For this review, take the finished solid that the model builds, in its own axes (mm). A direction names the side the tool comes from. Give positions to 0.01 mm unless a question says otherwise; leave off trailing zeros. Loops run counter-clockwise (first coordinate to the right, second up) from the corner with the lowest first, then second, coordinate; pieces in that order, holes last. Notation, with made-up numbers: (49.5, 68.25) -> (71.5, 68.25) arc R29 ccw to (71.5, 100.25) -> close; hole circle Ø9 at (-2.75, 47). An arc over 180 degrees is marked (long way). One line per question, with ' | ' between items. Start each with the question number.
(1) Consider section A-A (y = -4). Write out the cut boundary in (x, z), and give its area (3 significant figures).
(2) Wall thickness on probe 1 along Z at (x, y) = (3.5, 1.5); probe 2 along Y at (x, z) = (-4, 4.5); probe 3 along X at (y, z) = (0.75, 12.25): over which ranges is each line inside the solid? List them lowest first.
(3) Consider section C-C (z = 14.5). Write out the cut boundary in (x, y), and give its area (3 significant figures).
(4) Insertion check: P1, Ø5, axis at x = -4, z = 4.5, coming from the -Y side; P2, Ø1, axis at x = 2, z = 2, coming from the +Y side; P3, Ø5, axis at y = -3, z = 7, coming from the -X side. Each pin has a flat end and moves straight along its axis. Give the tip position at first contact, or say it passes through.
(5) Consider section B-B (x = -4.5). Write out the cut boundary in (y, z), and give its area (3 significant figures).
(6) Consider section D-D (x = 0). Write out the cut boundary in (y, z), and give its area (3 significant figures).
(7) Draft analysis for pull direction Z (two halves, no side actions). For faces 1 (the flat face through (-0.1, -3.3, 5)), 2 (the flat face through (0, 0, 0)), 3 (the cylindrical face through (-7.4, 0, 1.5)), state which applies: +Z half, -Z half, draft (parallel to the pull), parting line (faces both ways), or undercut.
(8) Tool access review of faces 4 (the cylindrical face through (-3, 0, 7)), 5 (the flat face through (0, 0, 18)): name each direction out of +Z, -Z, +X, -X, +Y, -Y from which nothing blocks a thin tool from reaching the whole face with its end or side.
from build123d import *

# Parameters (mm, degrees)
SKETCH2_R           = 5
BOSS_EXTRUDE1_DEPTH = 5
SKETCH3_R           = 3
BOSS_EXTRUDE2_DEPTH = 5
SKETCH4_R           = 5
BOSS_EXTRUDE3_DEPTH = 8
SKETCH5_R           = 1
BOSS_EXTRUDE4_DEPTH = 10


with BuildPart() as part:
    # Sketch2 → Boss-Extrude1 (new body)
    with BuildSketch(Plane.XY):
        Circle(SKETCH2_R)
    extrude(amount=BOSS_EXTRUDE1_DEPTH)

    # Sketch3 → Boss-Extrude2 (add)
    with BuildSketch(Plane.XY.offset(5)):
        Circle(SKETCH3_R)
    extrude(amount=BOSS_EXTRUDE2_DEPTH)

    # Sketch4 → Boss-Extrude3 (add)
    with BuildSketch(Plane.XY.offset(10)):
        Circle(SKETCH4_R)
    extrude(amount=BOSS_EXTRUDE3_DEPTH)

    # Sketch5 → Boss-Extrude4 (add)
    with BuildSketch(Plane.ZY):
        with Locations((2.5, 0)):
            Circle(SKETCH5_R)
    extrude(amount=BOSS_EXTRUDE4_DEPTH)


solid = part.part
A:
1) outline: (-3, 0) -> (3, 0) -> (3, 5) -> (-3, 5) -> close; (-3, 10) -> (3, 10) -> (3, 18) -> (-3, 18) -> close | area: 78.0 mm^2
2) probe 1: z = 0 to 5, 10 to 18 | probe 2: y = -3 to 3 | probe 3: x = -4.94 to 4.94
3) outline: circle Ø10 at (0, 0) | area: 78.5 mm^2
4) P1: stops at y = -4.77 | P2: stops at y = 4.77 | P3: stops at x = -4.77
5) outline: (-2.18, 0) -> (2.18, 0) -> (2.18, 5) -> (-2.18, 5) -> close; (-2.18, 10) -> (2.18, 10) -> (2.18, 18) -> (-2.18, 18) -> close | area: 56.7 mm^2
6) outline: (-5, 0) -> (5, 0) -> (5, 5) -> (3, 5) -> (3, 10) -> (5, 10) -> (5, 18) -> (-5, 18) -> (-5, 10) -> (-3, 10) -> (-3, 5) -> (-5, 5) -> close | area: 160 mm^2
7) face 1: undercut | face 2: -Z half | face 3: parting line
8) face 4: none | face 5: +Z, +X, -X, +Y, -Y
